Autodesk Inventor part; units mm, degrees
ref_plane "YZ Plane" through (0, 0, 0) normal (1, 0, 0) x (0, 1, 0)
ref_plane "XZ Plane" through (0, 0, 0) normal (0, 1, 0) x (-1, 0, 0)
ref_plane "XY Plane" through (0, 0, 0) normal (0, 0, 1) x (1, 0, 0)
sketch "Boceto1" plane through (0, 0, 0) normal (0, 1, 0) x (-1, 0, 0)
  line L0 (6.1283, -21.2541) -> (6.1283, -85.7541)
  line L1 (6.1283, -85.7541) -> (-253.3717, -85.7541)
  line L2 (6.1283, -21.2541) -> (-253.3717, -21.2541)
  line L3 (-253.3717, -21.2541) -> (-253.3717, -85.7541)
  circle A0 centre (-127.3717, -61.2541) radius 4
  circle A1 centre (-10.3717, -61.2541) radius 4
  circle A2 centre (-84.3717, -76.7541) radius 2
  circle A3 centre (-84.3717, -45.7541) radius 2
  circle A4 centre (-53.3717, -76.7541) radius 2
  circle A5 centre (-53.3717, -45.7541) radius 2
  circle A6 centre (-28.8717, -53.2541) radius 3
  circle A7 centre (-173.3717, -67.7541) radius 3
  circle A8 centre (-173.3717, -39.2541) radius 3
  dimension "d0" = 64.5
  dimension "d22" = 8
  dimension "d23" = 8
  dimension "d65" = 4
  dimension "d66" = 4
  dimension "d67" = 4
  dimension "d68" = 4
  dimension "d69" = 31
  dimension "d70" = 31
  dimension "d71" = 31
  dimension "d72" = 31
  dimension "d109" = 117
  dimension "d110" = 259.5
  dimension "d111" = 126
  dimension "d112" = 6
  dimension "d113" = 32
  dimension "d114" = 35
  dimension "d115" = 6
  dimension "d116" = 6
  dimension "d117" = 18
  dimension "d118" = 18
  dimension "d119" = 80
  dimension "d120" = 80
  dimension "d127" = 40
  dimension "d128" = 40
extrude "Extrusion3" add sketch "Boceto1" along normal blind 12
sketch "Sketch2" plane through (0, 0, 0) normal (0, -1, 0) x (1, 0, 0)
  circle A0 centre (6.3717, -26.2541) radius 3
  circle A1 centre (31.3717, -26.2541) radius 3
  line L0 (-6.1283, -21.2541) -> (253.3717, -21.2541)
  line L1 (-6.1283, -85.7541) -> (-6.1283, -21.2541)
  point P0 (0, 0)
  point P1 (-7.1283, -20.7541)
  point P2 (261.8717, -20.7541)
  point P3 (-7.1283, -85.7541)
  dimension "d84" = 6
  dimension "d85" = 6
  dimension "d86" = 5
  dimension "d87" = 12.5
  dimension "d88" = 25
  dimension "d89" = 5
extrude "Extrusion4" cut sketch "Sketch2" against normal blind 19
sketch "Sketch3" plane through (0, 12, 0) normal (0, 1, 0) x (1, 0, 0)
  circle A0 centre (218.3717, 71.2541) radius 3
  circle A1 centre (238.3717, 71.2541) radius 3
  circle A2 centre (218.3717, 36.2541) radius 3
  circle A3 centre (238.3717, 36.2541) radius 3
  line L0 (253.3717, 85.7541) -> (-6.1283, 85.7541)
  line L1 (-6.1283, 21.2541) -> (253.3717, 21.2541)
  line L2 (253.3717, 21.2541) -> (253.3717, 85.7541)
  point P0 (-7.1283, 85.7541)
  point P1 (-7.1283, 20.7541)
  dimension "d92" = 6
  dimension "d93" = 6
  dimension "d94" = 6
  dimension "d95" = 6
  dimension "d97" = 15
  dimension "d98" = 15
  dimension "d99" = 15
  dimension "d100" = 20
  dimension "d101" = 20
  dimension "d103" = 15
  dimension "d130" = 35
  dimension "d131" = 35
extrude "Extrusion5" cut sketch "Sketch3" against normal blind 20
thread "Rosca1"
thread "Rosca2"
thread "Rosca3"
equation "\"d22\" = d23"
equation "\"d118\" = d117"
equation "\"d120\" = d119"
equation "\"d131\" = d130"
equation "\"d104\" = d100"
properties part number "Columna Derecha" material "Aluminio 6061"
Can you work these out from the model? Positions are in its coordinate system, mm. Give positions to 0.01 mm unless a question says otherwise; leave off trailing zeros. Use one line per item in the form item = value.
Item 1: Thinking about a two-plate mould opening in Z: for faces 1 (the flat face through (125, 12, -53)), 2 (the flat face through (122, 6, -85.754)), 3 (the cylindrical face through (27.259, 5.916, -55.784)), which applies, pulls with the +Z half, pulls with the -Z half, needs draft (parallel to the pull), parting line crosses it, or undercut?
Values follow:
face_1 = needs draft
face_2 = pulls with the -Z half
face_3 = undercut
Item 2: If we section it at A-A, the plane y = 3.75: Count the separate pieces of the cut face and the enclosed holes in it, and give its area (3 significant figures).
Values follow:
separate_pieces = 1
enclosed_holes = 15
area = 16,300 mm^2
Item 3: Will this pin go through, and if not, where does the flat tip stop? pin 1 Ø7 at (x, z) = (10.37, -61.25) entering from +Y.
Values follow:
pin_1 = through
Item 4: If I drill on line 1 along X through (y, z) = (3.75, -37); line 2 along X through (y, z) = (1.5, -62.5); line 3 along X through (y, z) = (3, -34), over which ranges is the centre line in solid material (lowest first)? Write a range as [from, to].
Values follow:
line_1 = [-6.13, 171.39], [175.35, 215.47], [221.28, 235.47], [241.28, 253.37]
line_2 = [-6.13, 6.57], [14.17, 123.57], [131.17, 253.37]
line_3 = [-6.13, 216.39], [220.35, 236.39], [240.35, 253.37]
